Build history of the part. All positions in model axes, mm. Give positions to 0.01 mm unless a question says otherwise; leave off trailing zeros. Order: outer loops, then holes, each group sorted by start corner. A loop starts at its lowest first (then second) coordinate and runs counter-clockwise, first axis right, second up. Notation, with made-up numbers: (-4.75, 88.5) -> (44.25, 88.5) arc R22 cw to (44.25, 104.5) -> close; hole circle Ø5 at (44.25, 8.5). An arc over 180 degrees is marked (long way). Use a Markdown table: item, result. Add a question column.
Autodesk Inventor part; units mm, degrees
ref_plane "YZ Plane" through (0, 0, 0) normal (1, 0, 0) x (0, 1, 0)
ref_plane "XZ Plane" through (0, 0, 0) normal (0, 1, 0) x (-1, 0, 0)
ref_plane "XY Plane" through (0, 0, 0) normal (0, 0, 1) x (1, 0, 0)
sketch "スケッチ1" plane through (0, 0, 0) normal (0, 0, 1) x (1, 0, 0)
  line L0 (0, 3.1754) -> (2.75, 1.5877)
  line L1 (2.75, 1.5877) -> (2.75, -1.5877)
  line L2 (2.75, -1.5877) -> (0, -3.1754)
  line L3 (0, -3.1754) -> (-2.75, -1.5877)
  line L4 (-2.75, -1.5877) -> (-2.75, 1.5877)
  line L5 (-2.75, 1.5877) -> (0, 3.1754)
  point P0 (0, 0)
  point P1 (0, 0)
  dimension "d0" = 5.5
extrude "押し出し1" add sketch "スケッチ1" along normal blind 10
sketch "スケッチ2" plane through (0, 0, 10) normal (0, 0, 1) x (1, 0, 0)
  circle A0 centre (0, 0) radius 1.5
  dimension "d3" = 3
extrude "押し出し2" add sketch "スケッチ2" along normal blind 6
thread "ねじ1"
sketch "スケッチ3" plane through (0, 0, 0) normal (0, 0, -1) x (-1, 0, 0)
  point P0 (0, 0)
hole "穴1" at (0, 0, 0) direction (0, 0, 1) diameter 2.459 depth 8.8 tip angle 118
properties part number "ステンレススペーサー（六角）_BSU-310" material "ステンレス鋼"
(1) Mould opens along Y. For faces 1 (the face through (0.748, -0.976, 4.462)), 2 (the face through (-1.3, -1.4, 10)), 3 (the face through (-1.5, -0.07, 12.96)) say: released by +Y, released by -Y, zero draft, split by the parting line, or undercut.
(2) Band-saw the part on B-B on x = 2.1. Give the cut face in (y, z), plus the area to 3 significant figures.
(3) Band-saw the part on A-A on z = 2.75. Give the cut face in (x, y), plus the area to 3 significant figures.
(4) Wall check: probe 1 along X at (y, z) = (0, 6.25); probe 2 along Z at (x, y) = (-0.15, 2); probe 3 along X at (y, z) = (1, 7.5). Give the ranges that are in metal, low to high.
(5) Band-saw the part on C-C on y = 2.5. Give the cut face in (x, z).
(6) Pin check, flat tips, straight feed: pin 1 Ø2 at (x, y) = (0, 0) entering from -Z; pin 2 Ø1.5 at (x, z) = (1.5, 6.5) entering from -Y. Stop position of each tip, or through.
Response:
| question | item | result |
|---|---|---|
| 1 | face 1 | undercut |
| 1 | face 2 | zero draft |
| 1 | face 3 | split by the parting line |
| 2 | outline | (-1.96, 0) -> (1.96, 0) -> (1.96, 10) -> (-1.96, 10) -> close |
| 2 | area | 39.3 mm² |
| 3 | outline | (-2.75, -1.59) -> (0, -3.18) -> (2.75, -1.59) -> (2.75, 1.59) -> (0, 3.18) -> (-2.75, 1.59) -> close; hole circle Ø2.46 at (0, 0) |
| 3 | area | 21.4 mm² |
| 4 | probe 1 | x = -2.75 to -1.23, 1.23 to 2.75 |
| 4 | probe 2 | z = 0 to 10 |
| 4 | probe 3 | x = -2.75 to -0.72, 0.72 to 2.75 |
| 5 | outline | (-1.17, 0) -> (1.17, 0) -> (1.17, 10) -> (-1.17, 10) -> close |
| 6 | pin 1 | stops at z = 8.94 |
| 6 | pin 2 | stops at y = -2.74 |
